Part model, mm, in its own coordinate system. A direction names the side the tool comes from. Coordinates: 2 decimals unless noted, no trailing zeros. Loops run counter-clockwise (first coordinate to the right, second up) from the corner with the lowest first, then second, coordinate; pieces in that order, holes last.
```python
from build123d import *

# Parameters (mm, degrees)
SKETCH1_R               = 4.064
BOSS_EXTRUDE1_DEPTH     = 35.052
SKETCH2_W               = 28.956
SKETCH2_H               = 40.132
CUT_EXTRUDE1_DEPTH      = 59.42
SKETCH3_R               = 4.064
CUT_EXTRUDE3_DEPTH      = 44.18
CUT_EXTRUDE3_DEPTH_BACK = 35.052


with BuildPart() as part:
    # Sketch1 → Boss-Extrude1 (new body)
    with BuildSketch(Plane(origin=(0, 0, 0), x_dir=(0, 0, -1), z_dir=(1, 0, 0))):
        with BuildLine():
            Line((0, 16.002), (45.896514256, 42.085387724))
            ThreePointArc((45.896514256, 42.085387724), (54.253684434, 42.0427173), (58.42, 34.798))
            Line((58.42, 34.798), (58.42, 0))
            Line((58.42, 0), (0, 0))
            Line((0, 0), (0, 16.002))
        make_face()
        with Locations((50.038, 34.798)):
            Circle(SKETCH1_R, mode=Mode.SUBTRACT)
    extrude(amount=-BOSS_EXTRUDE1_DEPTH)

    # Sketch2 → Cut-Extrude1 (cut, through all)
    with BuildSketch(Plane.XY):
        with Locations((-17.526, 23.114)):
            Rectangle(SKETCH2_W, SKETCH2_H)
    extrude(amount=-CUT_EXTRUDE1_DEPTH, mode=Mode.SUBTRACT)

    # Sketch3 → Cut-Extrude3 (cut, two sides)
    with BuildSketch(Plane(origin=(0, 0, 0), x_dir=(1, 0, 0), z_dir=(0, 1, 0))) as cut_extrude3_sk:
        with Locations(Location((-17.526, 12.446, 0), (0, 0, 90))):  # turned: the seam where the file's is
            Circle(SKETCH3_R)
        with BuildLine():
            Line((-21.844, 43.930247399), (-21.844, 58.42))
            Line((-21.844, 58.42), (-13.208, 58.42))
            Line((-13.208, 58.42), (-13.208, 43.930247399))
            ThreePointArc((-13.208, 43.930247399), (-17.526, 39.612247399), (-21.844, 43.930247399))
        make_face()
    extrude(amount=CUT_EXTRUDE3_DEPTH, mode=Mode.SUBTRACT)
    extrude(cut_extrude3_sk.sketch, amount=-CUT_EXTRUDE3_DEPTH_BACK, mode=Mode.SUBTRACT)


solid = part.part
```
Q1. Mould opens along Z. For faces 4 (the flat face through (-32.3, 14.9, -58.42)), 5 (the flat face through (-21.844, 2, -51)), 6 (the cylindrical face through (-13.92, 1.5, -14.32)) say: released by +Z, released by -Z, zero draft, split by the parting line, or undercut.
Q2. Saw through at C-C (z = -11). List the corners of the cut face in (x, y).
Q3. Tool access for faces 1 (the flat face through (-3.048, 18, -35)), 2 (the flat face through (-13.208, 2, -51)), 3 (the flat face through (-1.503, 28.861, -22.627)): list every direction of +Z, -Z, +X, -X, +Y, -Y with a clear straight run to the whole face (end or side of a thin tool).
Q4. Saw through at D-D (z = -28). List the corners of the cut face in (x, y), plus the area to 3 significant figures.
Q5. Saw through at A-A (y = 14). List the corners of the cut face in (x, z).
Q6. Drop flat-ended pins along their axis: P1, Ø10.5, axis at y = 34.798, z = -50.038, coming from the -X side; P2, Ø10.5, axis at x = -17.526, z = -12.446, coming from the +Y side. Give the stop position or say it passes through.
Q7. Probe line 1 (X direction, y = 9.5, z = -10); line 2 (Y direction, x = -12, z = -20); line 3 (Z direction, x = -3, y = 19). List the from-to ranges inside material, lowest first.
Q8. Saw through at B-B (x = -15). List the corners of the cut face in (y, z), plus the area to 3 significant figures.
Checked values:
1. face 4: released by -Z
1. face 5: zero draft
1. face 6: undercut
2. outline: (-35.05, 0) - (-21.32, 0) - (-21.32, 3.05) - (-32, 3.05) - (-32, 22.25) - (-35.05, 22.25) - close; (-13.73, 0) - (0, 0) - (0, 22.25) - (-3.05, 22.25) - (-3.05, 3.05) - (-13.73, 3.05) - close
3. face 1: +Z, -Z, +Y
3. face 2: -Z, +Y, -Y
3. face 3: +Z, +X, -X, +Y
4. outline: (-35.05, 0) - (0, 0) - (0, 31.91) - (-3.05, 31.91) - (-3.05, 3.05) - (-32, 3.05) - (-32, 31.91) - (-35.05, 31.91) - close
4. area: 283 mm2
5. outline: (-35.05, -58.42) - (-32, -58.42) - (-32, 0) - (-35.05, 0) - close; (-3.05, -58.42) - (0, -58.42) - (0, 0) - (-3.05, 0) - close
6. P1: stops at x = -35.05
6. P2: stops at y = 3.05
7. line 1: x = -35.05 to -32, -3.05 to 0
7. line 2: y = 0 to 3.05
7. line 3: z = -58.42 to -5.28
8. outline: (0, -40.43) - (3.05, -40.43) - (3.05, -15.63) - (0, -15.63) - close; (0, -9.26) - (3.05, -9.26) - (3.05, 0) - (0, 0) - close
8. area: 104 mm2
